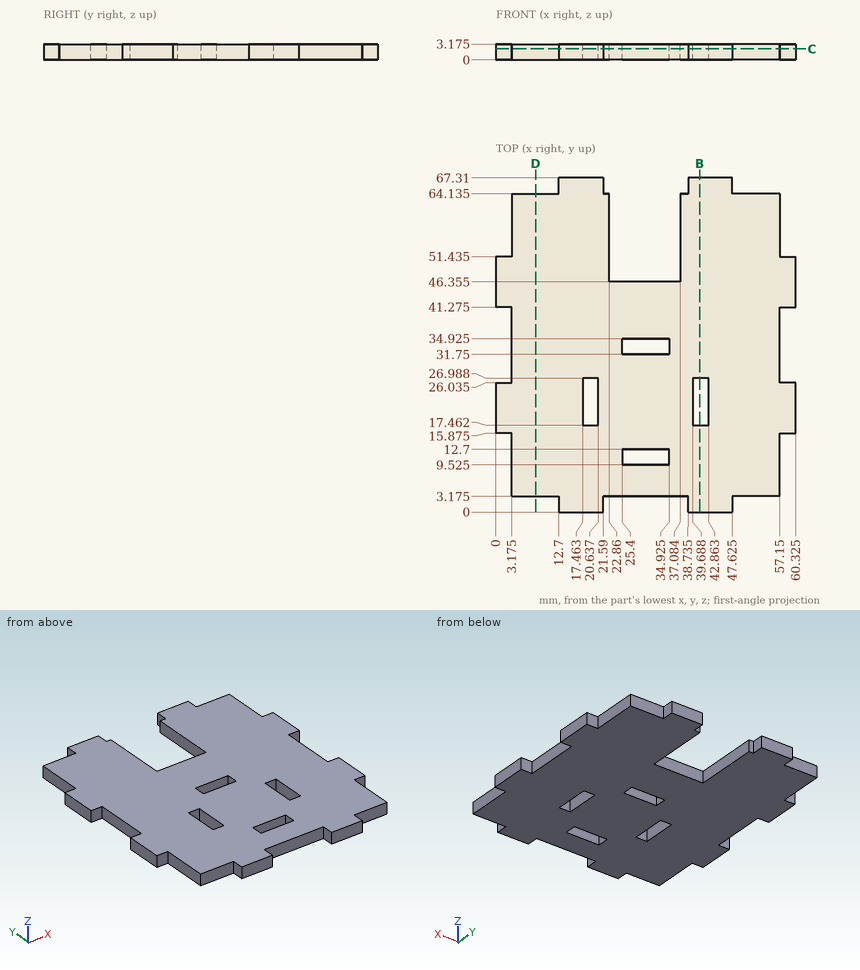
The figure shows three views and two pictorial views of one solid part (mm, origin at its lowest corner). Answer the questions. Coordinates: 2 decimals unless noted, no trailing zeros. Loops run counter-clockwise (first coordinate to the right, second up) from the corner with the lowest first, then second, coordinate; pieces in that order, holes last. Notation, with made-up numbers: (43, 0) -> (84, 0) arc R27 ccw to (84, 31) -> close; hole circle Ø1 at (-28.75, 31). An arc over 180 degrees is marked (long way). Write item = value, one per line. Start each with the question number.
1) A cutting plane is placed at B-B (x = 41). Give the vertices of the cut face in (y, z) (1 decimal).
2) A cutting plane is placed at D-D (x = 8). Give the vertices of the cut face in (y, z) (1 decimal).
3) Given pin 1 Ø1.6 at (x, z) = (29.5, 2) entering from -Y (1 decimal); pin 2 Ø1 at (y, z) = (34, 2.5) entering from +X; pin 3 Ø1 at (x, z) = (1, 2) entering from +Y (1 decimal); pin 4 Ø6 at (x, y) = (28.5, 52.5) entering from -Z, each flat-ended and moving along its own axis, determine where each tip first touches the part or whether it passes through.
4) Straight lines are drawn through the part: line 1 (X direction, y = 24.5, z = 1.3) (1 decimal); line 2 (X direction, y = 3, z = 0.4) (1 decimal); line 3 (X direction, y = 50, z = 2.7) (1 decimal). For each, find the intervals that lie inside material, in ascending order. Write a range as from..to.
5) A cutting plane is placed at C-C (z = 2.2). Count the separate pieces of the cut face and the enclosed holes in it, then the cut area to 3 significant figures.
Responses:
q1.outline = (0, 0) -> (17.5, 0) -> (17.5, 3.2) -> (0, 3.2) -> close; (27, 0) -> (67.3, 0) -> (67.3, 3.2) -> (27, 3.2) -> close
q2.outline = (3.2, 0) -> (64.1, 0) -> (64.1, 3.2) -> (3.2, 3.2) -> close
q3.pin_1 = 3.2
q3.pin_2 = 57.15
q3.pin_3 = 51.4
q3.pin_4 = through
q4.line_1 = 0..17.5, 20.6..39.7, 42.9..60.3
q4.line_2 = 12.7..21.6, 38.7..47.6
q4.line_3 = 0..22.9, 37.1..60.3
q5.separate_pieces = 1
q5.enclosed_holes = 4
q5.area = 3,160 mm²
